from build123d import *

# Parameters (mm, degrees)
SKETCH8_R           = 2
SKETCH8_R_2         = 1.5
BOSS_EXTRUDE3_DEPTH = 3
BOSS_EXTRUDE4_DEPTH = 5


with BuildPart() as part:
    # Sketch8 → Boss-Extrude3 (new body)
    # profile 1 of 2: a face of its own
    with BuildSketch(Plane(origin=(0, 0, 0), x_dir=(0, 0, -1), z_dir=(1, 0, 0))):
        with BuildLine():
            ThreePointArc((13.132863069, 0.320027848), (3.75419069, 5.150346209), (-5.956033277, 1.026874177))
            Line((-5.956033277, 1.026874177), (-4.319797484, 1.050447619))
            ThreePointArc((-4.319797484, 1.050447619), (4.590085283, 3.936033014), (12.605766771, -0.907670556))
            Line((12.605766771, -0.907670556), (13.12184584, -1.999779955))
            Line((13.12184584, -1.999779955), (14.377901927, -6.177963459))
            ThreePointArc((14.377901927, -6.177963459), (15.022692005, -4.057588727), (17.227616297, -3.83386543))
            ThreePointArc((17.227616297, -3.83386543), (14.859483295, -2.073108487), (13.132863069, 0.320027848))
        make_face()
    # profile 2 of 2: a face of its own
    with BuildSketch(Plane(origin=(0, 0, 0), x_dir=(0, 0, -1), z_dir=(1, 0, 0))):
        with Locations((16.293226017, -5.602173889)):
            Circle(SKETCH8_R)
        with Locations((16.293226017, -5.602173889)):
            Circle(SKETCH8_R_2, mode=Mode.SUBTRACT)
    extrude(amount=BOSS_EXTRUDE3_DEPTH)

    # Sketch10 → Boss-Extrude4 (add)
    with BuildSketch(Plane(origin=(3, 0, 0), x_dir=(0, 0, -1), z_dir=(1, 0, 0))):
        with BuildLine():
            Line((-5.956033277, 1.026874177), (-4.319797484, 1.050447619))
            ThreePointArc((-4.319797484, 1.050447619), (-2.522150549, 2.39412043), (-0.493946712, 3.355047235))
            Line((-0.493946712, 3.355047235), (-1.051379481, 4.37374771))
            ThreePointArc((-1.051379481, 4.37374771), (-3.706640914, 2.997700023), (-5.956033277, 1.026874177))
        make_face()
    extrude(amount=BOSS_EXTRUDE4_DEPTH)


solid = part.part
Read the model definition and answer for the solid it produces. Units are mm, in the model's axes. Round coordinates to 2 decimals unless told otherwise and drop trailing zeros. Order: outer loops, then holes, each group sorted by start corner. A loop starts at its lowest first (then second) coordinate and runs counter-clockwise, first axis right, second up.
1) The part is cut by section D-D on y = -6.5. Write down the section's boundary in (x, z), plus the area to 3 significant figures.
2) The part is cut by section C-C on x = 7.5. Write down the section's boundary in (y, z).
3) The part is cut by section A-A on y = 2. Write down the section's boundary in (x, z), plus the area to 3 significant figures.
4) The part is cut by section B-B on x = 2.5. Write down the section's boundary in (y, z).
5) Straight lines are drawn through the part: L1, parallel to Z at x = 2.75, y = 2.5; L2, parallel to Z at x = 0.75, y = -4.75; L3, parallel to Y at x = 1.5, z = -9.5. For each, find the intervals that lie inside material, in ascending order.
6) Flat-ended cylindrical pins translate along their axes: pin 1 (1.5 mm diameter, centred on x = 3, z = -1.5, fed in from +Y); pin 2 (4 mm diameter, centred on x = 5.5, y = 3.5, fed in from +Z). Find the tip coordinate at first contact, or state that the pin passes through.
7) The mould has two halves that part along Z. Classify faces 1 (the face through (1.48, -1.45, -12.86)), 2 (the face through (5.46, 3.86, 0.77)), 3 (the face through (1.479, -5.152, -17.724)), 4 (the face through (1.48, -7.18, -17.52)): released by +Z, released by -Z, zero draft, split by the parting line, or undercut.
Resolved:
1. outline: (0, -18.08) - (3, -18.08) - (3, -17.49) - (0, -17.49) - close; (0, -15.09) - (3, -15.09) - (3, -14.51) - (0, -14.51) - close
1. area: 3.51 mm2
2. outline: (1.03, 5.96) - (1.05, 4.32) arc R11.27 cw to (3.36, 0.49) - (4.37, 1.05) arc R12.42 ccw to start
3. outline: (0, -11.57) - (3, -11.57) - (3, -9.72) - (0, -9.72) - close; (0, 3.13) - (8, 3.13) - (8, 4.98) - (0, 4.98) - close
3. area: 20.4 mm2
4. outline: (-6.18, -14.38) arc R2 ccw (long way) to (-3.83, -17.23) arc R9.67 cw to (0.32, -13.13) arc R12.42 ccw to (1.03, 5.96) - (1.05, 4.32) arc R11.27 cw to (-0.91, -12.61) - (-2, -13.12) - close; hole circle Ø3 at (-5.6, -16.29)
5. L1: z = -10.97 to -8.93, 2.34 to 4.39
5. L2: z = -18.1 to -17.53, -15.06 to -13.95
5. L3: y = 2.15 to 3.5
6. pin 1: stops at y = 5.11
6. pin 2: stops at z = 5.51
7. face 1: released by +Z
7. face 2: released by -Z
7. face 3: undercut
7. face 4: split by the parting line
